Input: dimensioned drawing with shaded views. Units: mm. Origin: part minimum x, y, z. Coordinates: 2 decimals unless noted, no trailing zeros. Loops run counter-clockwise (first coordinate to the right, second up) from the corner with the lowest first, then second, coordinate; pieces in that order, holes last. Notation, with made-up numbers: (14.25, 62.5) - (58.25, 62.5) arc R12 ccw to (58.25, 84.5) - close; hole circle Ø2 at (-29.5, 24). An arc over 180 degrees is marked (long way). Write item = value, one per line. Start each with the question number.
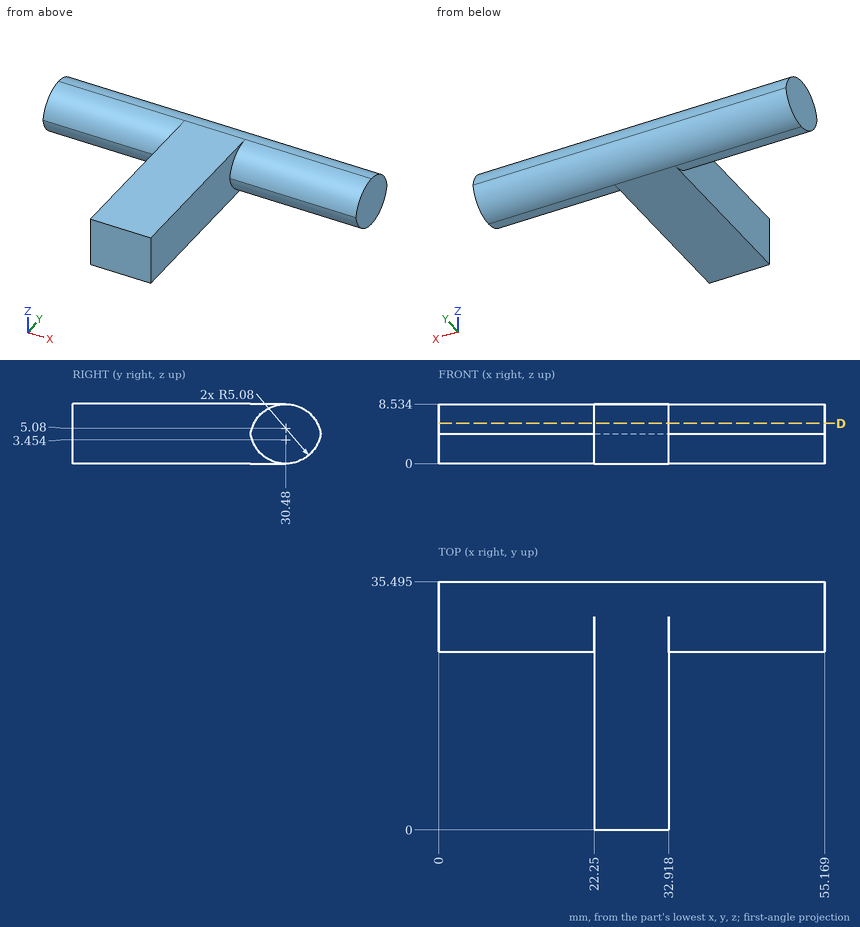
Item 1: Cut plane D-D on z = 5.75. Return loops of the section in (x, y).
Item 2: Ray query, line 1 (X direction, y = 5.5, z = 4.75); line 2 (Y direction, x = 21, z = 3) (1 decimal); line 3 (Y direction, x = 28.5, z = 3.25). Return the intervals inside material, ascending.
Item 3: Pin query (flat end, axial travel): pin 1 (4 mm diameter, centred on y = 11.5, z = 3.5, fed in from -X); pin 2 (1 mm diameter, centred on x = 48, z = 6.5, fed in from -Y) (1 decimal); pin 3 (4 mm diameter, centred on x = 12, y = 28, fed in from +Z). Return the tip coordinate at first contact, or that it passes through.
Recorded:
q1.outline = (0, 25.95) - (22.25, 25.95) - (22.25, 0) - (32.92, 0) - (32.92, 25.95) - (55.17, 25.95) - (55.17, 35.01) - (0, 35.01) - close
q2.line_1 = 22.25 to 32.92
q2.line_2 = 25.8 to 35.1
q2.line_3 = 0 to 35.22
q3.pin_1 = 22.25
q3.pin_2 = 26.1
q3.pin_3 = 8.51
